Design review of the part built by this model. Coordinates are the model's own, in mm. Coordinates: 2 decimals unless noted, no trailing zeros. Order: outer loops, then holes, each group sorted by start corner. A loop starts at its lowest first (then second) coordinate and runs counter-clockwise, first axis right, second up. Notation, with made-up numbers: M -34,60.5 L 17,60.5 A13 ccw 17,72.5 Z; hole C 23,85 d5. An arc over 180 degrees is marked long. Answer as a JSON object with one key per item and string values.
Autodesk Inventor part; units mm, degrees
ref_plane "YZ Plane" through (0, 0, 0) normal (1, 0, 0) x (0, 1, 0)
ref_plane "XZ Plane" through (0, 0, 0) normal (0, 1, 0) x (-1, 0, 0)
ref_plane "XY Plane" through (0, 0, 0) normal (0, 0, 1) x (1, 0, 0)
sketch "Sketch2" plane through (0, 0, 0) normal (0, 0, 1) x (1, 0, 0)
  circle A0 centre (-43, -20) radius 2.067
  circle A1 centre (-143, -20) radius 2.067
  circle A2 centre (-93, 20) radius 2.067
  circle A3 centre (-193, -20) radius 2.067
  circle A4 centre (20, 0) radius 2.067
  circle A5 centre (0, 20) radius 2.067
  circle A6 centre (-193, 20) radius 2.067
  circle A7 centre (-143, 20) radius 2.067
  circle A8 centre (-43, 20) radius 2.067
  circle A9 centre (-93, -20) radius 2.067
  circle A10 centre (0, -20) radius 2.067
  line L0 (-195.5, -22.5) -> (-195.5, 22.5)
  line L1 (-195.5, -22.5) -> (0, -22.5)
  arc A11 (0, -22.5) -> (0, 22.5) centre (0, 0) ccw
  line L2 (-195.5, 22.5) -> (0, 22.5)
  line L3 (0, -17.5) -> (-190.5, -17.5)
  line L4 (-190.5, -17.5) -> (-190.5, 17.5)
  line L5 (-190.5, 17.5) -> (0, 17.5)
  arc A12 (0, -17.5) -> (0, 17.5) centre (0, 0) ccw
  point P0 (-197.5, 0)
extrude "Extrusion1" add sketch "Sketch2" along normal mid plane 10 contours L0 L2 A11 L1 | L3 L4 L5 A12
chamfer "Chamfer1" distance 10 angle 45 3 edges at (-97.75, 22.5, 5) (22.5, 0, 5) (-97.75, -22.5, 5)
fillet "Fillet2" radius 10 3 edges at (-97.75, -12.5, 5) (12.5, 0, 5) (-97.75, 12.5, 5)
properties part number "Cover for robot head" material "Steel, Alloy"
1) Add section A-A (x = -93). State the section outline as (y, z) points.
Taken from the geometry:
{"outline": "M -22.5,-5 L -22.07,-5 L -22.07,-4.57 Z; M -17.93,-5 L 17.93,-5 L 17.93,-0.43 L 15.43,2.07 A10 ccw 8.36,5 L -8.36,5 A10 ccw -15.43,2.07 L -17.93,-0.43 Z; M 22.07,-5 L 22.5,-5 L 22.07,-4.57 Z"}
2) Mouldability with a two-part tool opening along X and no side actions: class faces 1 (the cylindrical face through (-193.448, 17.982, -3.189)), 2 (the cylindrical face through (-93.448, 17.982, -3.189)), 3 (the flat face through (-99.1, 19, -1.5)), 4 (the flat face through (-195.5, 0, 0)) as released by +X, released by -X, zero draft, split by the parting line, or undercut.
Taken from the geometry:
{"face 1": "undercut", "face 2": "undercut", "face 3": "zero draft", "face 4": "released by -X"}
3) Add section C-C (y = 20). Count the separate pieces of the cut face and the enclosed holes in it, and give its area (3 significant figures).
Taken from the geometry:
{"separate pieces": "6", "enclosed holes": "0", "area": "454 mm2"}
4) Insertion check: pin 1 Ø6.5 at (x, y) = (-43, -20) entering from +Z; pin 2 Ø5.5 at (x, y) = (-193, -20) entering from -Z; pin 3 Ø1 at (x, y) = (-151, 9.5) entering from +Z; pin 4 Ø5.5 at (x, y) = (-143, 20) entering from +Z. Each pin has a flat end and moves straight along its axis. Give the tip position at first contact, or say it passes through.
Taken from the geometry:
{"pin 1": "stops at z = 0.75", "pin 2": "stops at z = -5", "pin 3": "stops at z = 4.98", "pin 4": "stops at z = 0.25"}
5) To check wall thickness, follow L1, parallel to Y at x = 0, z = -3.85; L2, parallel to Z at x = -73, y = 14.5; L3, parallel to Y at x = -181, z = 1. State the ranges of each line that lie inside material, in increasing order.
Taken from the geometry:
{"L1": "y = -17.93 to 17.93", "L2": "z = -5 to 2.89", "L3": "y = -16.5 to 16.5"}
6) Add section B-B (x = -157). State the section outline as (y, z) points.
Taken from the geometry:
{"outline": "M -22.5,-5 L 22.5,-5 L 15.43,2.07 A10 ccw 8.36,5 L -8.36,5 A10 ccw -15.43,2.07 Z"}
